from build123d import *

# Parameters (mm, degrees)
CROQUIS1_W              = 22.8
CROQUIS1_H              = 24
SALIENTE_EXTRUIR2_DEPTH = 11.6
CROQUIS2_R              = 2.5
SALIENTE_EXTRUIR3_DEPTH = 2


with BuildPart() as part:
    # Croquis1 → Saliente-Extruir2 (new body)
    with BuildSketch(Plane.XY):
        with Locations((0, 12)):
            Rectangle(CROQUIS1_W, CROQUIS1_H)
    extrude(amount=SALIENTE_EXTRUIR2_DEPTH)

    # Croquis2 → Saliente-Extruir3 (add)
    # profile 1 of 2: a face of its own
    with BuildSketch(Plane.XZ):
        with BuildLine():
            ThreePointArc((-5.7, 11.3), (-0.2, 5.8), (-5.7, 0.3))
            add(Edge.make_bspline(
                [(-13.4, 54.6), (-33.650343632, 14.235003165), (-5.7, 0.3)],
                knots=[0, 0, 0, 1, 1, 1], degree=2))
            add(Edge.make_bspline(
                [(-10.4, 51.6), (-14.231568326, 50.359614524), (-13.4, 54.6)],
                knots=[0, 0, 0, 1, 1, 1], degree=2))
            add(Edge.make_bspline(
                [(-5.7, 11.3), (-25.29034591, 18.195219879), (-10.4, 51.6)],
                knots=[0, 0, 0, 1, 1, 1], degree=2))
        make_face()
        with Locations(Location((-5.7, 5.8, 0), (0, 0, 270))):
            Circle(CROQUIS2_R, mode=Mode.SUBTRACT)
    # profile 2 of 2: a face of its own
    with BuildSketch(Plane.XZ):
        with BuildLine():
            ThreePointArc((5.7, 11.3), (0.2, 5.8), (5.7, 0.3))
            add(Edge.make_bspline(
                [(13.4, 54.6), (33.650343632, 14.235003165), (5.7, 0.3)],
                knots=[0, 0, 0, 1, 1, 1], degree=2))
            add(Edge.make_bspline(
                [(10.4, 51.6), (14.231568326, 50.359614524), (13.4, 54.6)],
                knots=[0, 0, 0, 1, 1, 1], degree=2))
            add(Edge.make_bspline(
                [(5.7, 11.3), (25.29034591, 18.195219879), (10.4, 51.6)],
                knots=[0, 0, 0, 1, 1, 1], degree=2))
        make_face()
        with Locations(Location((5.7, 5.8, 0), (0, 0, 90))):
            Circle(CROQUIS2_R, mode=Mode.SUBTRACT)
    extrude(amount=SALIENTE_EXTRUIR3_DEPTH)


solid = part.part
Verification items for the finished model (mm, model axes). A direction names the side the tool comes from. Coordinates: 2 decimals unless noted, no trailing zeros. Order: outer loops, then holes, each group sorted by start corner. A loop starts at its lowest first (then second) coordinate and runs counter-clockwise, first axis right, second up.
Item 1: Material ranges on L1, parallel to X at y = -0.8, z = 5.8; L2, parallel to Z at x = 4, y = 21.5; L3, parallel to X at y = 19.75, z = 3, recorded low to high.
Filled in:
L1: x = -13.81 to -8.2, -3.2 to -0.2, 0.2 to 3.2, 8.2 to 13.81
L2: z = 0 to 11.6
L3: x = -11.4 to 11.4
Item 2: Depth check by flat-ended pin: pin 1 (4.5 mm diameter, centred on x = 16.5, z = 21.5, fed in from +Y); pin 2 (7 mm diameter, centred on x = -3, y = 14, fed in from +Z); pin 3 (3.5 mm diameter, centred on y = 11.5, z = 8.5, fed in from -X). Enter the tip coordinate at first touch or a pass-through.
Filled in:
pin 1: stops at y = 0
pin 2: stops at z = 11.6
pin 3: stops at x = -11.4
Item 3: Access from +Z, -Z, +X, -X, +Y, -Y to the whole of each face (thin tool, end or side, straight path). Record for faces 1 (the face through (11.4, 12, 6)), 2 (the face through (17, -2, 20)), 3 (the face through (0, 12, 0)), 4 (the face through (-11.4, 12, 6)), 5 (the face through (0, 0, 4)).
Filled in:
face 1: +Z, -Z, +X, +Y
face 2: +Z, -Z, +X, -X, -Y
face 3: -Z, +X, -X, +Y, -Y
face 4: +Z, -Z, -X, +Y
face 5: -Y
Item 4: Section check A-A, the plane y = 18. Enter the section's corners in (x, z), then the cut area to 3 significant figures.
Filled in:
outline: (-11.4, 0) - (11.4, 0) - (11.4, 11.6) - (-11.4, 11.6) - close
area: 264 mm2
Item 5: Release check for a two-part mould opening along Z. For faces 6 (the face through (17, 0, 27)), 7 (the face through (0.2, -1, 5.9)), 8 (the face through (6, 0, 6)), 9 (the face through (0, 12, 11.6)) record: +Z half, -Z half, draft (parallel to the pull), parting line (faces both ways), or undercut.
Filled in:
face 6: draft
face 7: parting line
face 8: undercut
face 9: +Z half
